Geometry check sheet. Reference: the model listing, model coordinates, mm. Face numbers are marked on the shaded views. A direction names the side the tool comes from. Round coordinates to 2 decimals unless told otherwise and drop trailing zeros. Loops run counter-clockwise (first coordinate to the right, second up) from the corner with the lowest first, then second, coordinate; pieces in that order, holes last. Notation, with made-up numbers: M -3.75,28 L 49.25,28 A23 cw 49.25,49 Z; hole C -0.75,34 d5. An arc over 180 degrees is marked long. Write item = value, one per line.
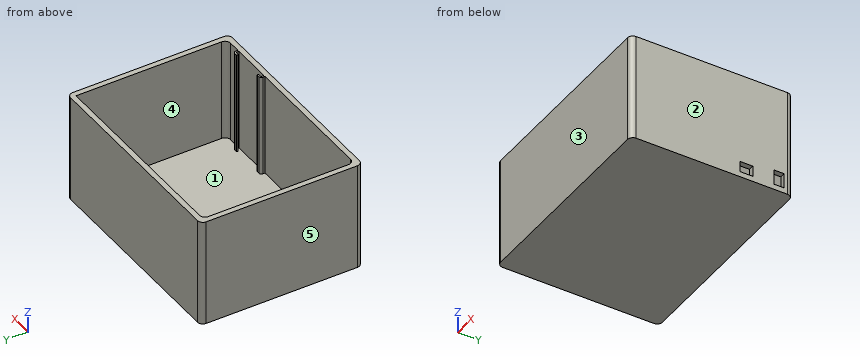
Solid Edge part; units mm, degrees
sketch "Sketch1" plane through (0, 0, 0) normal (0, 0, 1) x (1, 0, 0)
  line L0 (-100, -75) -> (100, -75)
  line L1 (100, -75) -> (100, 75)
  line L2 (100, 75) -> (-100, 75)
  line L3 (-100, 75) -> (-100, -75)
extrude "Protrusion1" add sketch "Sketch1" along normal blind 100
shell "Parede" thickness 5 removed faces 1 at (-68.6667, -48.5, 100)
sketch "Sketch2" plane through (100, 0, 50) normal (1, 0, 0) x (0, 0, -1)
  line L0 (45, 67.0982) -> (31, 67.0982)
  line L1 (31, 67.0982) -> (31, 57.5982)
  line L2 (31, 57.5982) -> (45, 57.5982)
  line L3 (45, 67.0982) -> (45, 57.5982)
  line L4 (45, 37.9671) -> (45, 25.9671)
  line L5 (35, 25.9671) -> (45, 25.9671)
  line L6 (35, 37.9671) -> (35, 25.9671)
  line L7 (45, 37.9671) -> (35, 37.9671)
extrude "Cutout1" cut sketch "Sketch2" against normal up to next
sketch "Sketch3" plane through (2.5, 0, 5) normal (0, 0, 1) x (1, 0, 0)
  line L0 (25.4753, 67.2334) -> (25.4753, 70)
  line L1 (23.4753, 70) -> (25.4753, 70)
  line L2 (23.4753, 68.092) -> (23.4753, 70)
  line L3 (21.1849, 65.9162) -> (23.4753, 68.092)
  line L4 (21.1849, 30.6261) -> (21.1849, 65.9162)
  line L5 (23.4753, 28.2151) -> (21.1849, 30.6261)
  line L6 (23.4753, 16.8218) -> (23.4753, 28.2151)
  line L7 (26.002, 13.874) -> (23.4753, 16.8218)
  line L8 (92.5, 13.874) -> (26.002, 13.874)
  line L9 (92.5, 15.874) -> (92.5, 13.874)
  line L10 (92.5, 15.874) -> (26.9219, 15.874)
  line L11 (26.9219, 15.874) -> (25.4753, 17.5616)
  line L12 (25.4753, 17.5616) -> (25.4753, 29.0137)
  line L13 (25.4753, 29.0137) -> (23.1849, 31.4246)
  line L14 (23.1849, 31.4246) -> (23.1849, 65.0575)
  line L15 (23.1849, 65.0575) -> (25.4753, 67.2334)
  circle A0 centre (25.4753, 62.4055) radius 1.3122
  circle A1 centre (25.4753, 34.1973) radius 1.3122
  circle A2 centre (76.8288, 18.8877) radius 1.3122
extrude "Parede_Arduino" add sketch "Sketch3" along normal blind 10
fillet "Round_1" radius 5 7 edges at (-100, -75, 50) (100, -75, 50) (100, 75, 50) (-100, 75, 50) (-95, -70, 52.5) (-95, 70, 52.5) (95, -70, 52.5)
sketch "Sketch4" plane through (0, 0, 5) normal (0, 0, 1) x (-1, 0, 0)
  line L0 (-38.2665, 70) -> (-38.2665, 68.0013)
  arc A0 (-40.5165, 65.7513) -> (-38.2665, 68.0013) centre (-40.5165, 68.0013) ccw
  line L1 (-40.5165, 65.7513) -> (-42.8072, 65.7513)
  arc A1 (-42.8072, 65.7513) -> (-42.8072, 67.2513) centre (-42.8072, 66.5013) cw
  line L2 (-40.5165, 67.2513) -> (-42.8072, 67.2513)
  arc A2 (-39.7665, 68.0013) -> (-40.5165, 67.2513) centre (-40.5165, 68.0013) cw
  line L3 (-39.7665, 70) -> (-39.7665, 68.0013)
  line L4 (-39.7665, 70) -> (-38.2665, 70)
  line L5 (-77.2665, 70) -> (-77.2665, 68.0013)
  arc A3 (-76.5165, 67.2513) -> (-77.2665, 68.0013) centre (-76.5165, 68.0013) cw
  line L6 (-76.5165, 67.2513) -> (-74.2258, 67.2513)
  arc A4 (-74.2258, 67.2513) -> (-74.2258, 65.7513) centre (-74.2258, 66.5013) cw
  line L7 (-76.5165, 65.7513) -> (-74.2258, 65.7513)
  arc A5 (-78.7665, 68.0013) -> (-76.5165, 65.7513) centre (-76.5165, 68.0013) ccw
  line L8 (-78.7665, 70) -> (-78.7665, 68.0013)
  line L9 (-78.7665, 70) -> (-77.2665, 70)
extrude "Protrusion2" add sketch "Sketch4" along normal up to vertex (95 mm away)
(1) Tool access check on the marked faces 4 and 5. Record the directions out of +Z, -Z, +X, -X, +Y, -Y that give a thin tool (end or side, any length) a straight path to the whole face; none if there is none.
Result set:
face_4 = +Z
face_5 = +Z, -Z, -X, +Y, -Y
(2) Sectioned sample at B-B on y = -30. Record the cut outline in (x, z), then the cut area to 3 significant figures.
Result set:
outline = M -100,0 L 100,0 L 100,100 L 95,100 L 95,5 L -95,5 L -95,100 L -100,100 Z
area = 1,950 mm2
(3) Sectioned sample at C-C on x = -66.5. Record the cut outline in (y, z), then the cut area to 3 significant figures.
Result set:
outline = M -75,0 L 75,0 L 75,100 L 70,100 L 70,5 L -70,5 L -70,100 L -75,100 Z
area = 1,700 mm2
(4) Release check for a two-part mould opening along Y. For the marked faces 1, 2 and 3 record: released by +Y, released by -Y, zero draft, split by the parting line, or undercut.
Result set:
face_1 = undercut
face_2 = zero draft
face_3 = released by -Y
(5) Depth check by flat-ended pin: pin 1 Ø5.5 at (x, z) = (98.5, 8.5) entering from -Y; pin 2 Ø1 at (x, y) = (8.5, 11) entering from +Z; pin 3 Ø0.8 at (x, y) = (28.5, 62.5) entering from +Z. Enter the tip coordinate at first touch or a pass-through.
Result set:
pin_1 = -74.94
pin_2 = 5
pin_3 = 15
(6) Material ranges on line 1 along X through (y, z) = (-60.5, 37); line 2 along Y through (x, z) = (-85, 66); line 3 along Z through (x, y) = (-10, -16), recorded low to high. Write a range as from..to.
Result set:
line_1 = -100..-95, 95..100
line_2 = -75..-70, 70..75
line_3 = 0..5
